The model under review builds one solid part; all positions refer to its coordinate system, in mm. A direction names the side the tool comes from. Round coordinates to 2 decimals unless told otherwise and drop trailing zeros. Order: outer loops, then holes, each group sorted by start corner. A loop starts at its lowest first (then second) coordinate and runs counter-clockwise, first axis right, second up.
1) To check wall thickness, follow L1, parallel to Z at x = 5.75, y = 24 (3 decimals); L2, parallel to X at y = 8, z = -2.5. State the ranges of each line that lie inside material, in increasing order.
2) Consider section D-D (y = 18.5). Give the boundary of the cut face in (x, z) (3 decimals).
3) Consider section B-B (x = 9). Give the boundary of the cut face in (y, z) (3 decimals), then the cut area to 3 significant figures.
4) Consider section A-A (y = 30). Give the boundary of the cut face in (x, z) (3 decimals), then the cut area to 3 significant figures.
5) Machinability: for faces 4 (the face through (0, 23, -24)), 5 (the face through (-1.565, 19.482, -37.514)), which of the approach directions +Z, -Z, +X, -X, +Y, -Y give a long, thin tool a straight path to every point of the face, cutting with its end or side? Answer none if there is none.
6) Consider section C-C (x = -2). Give the boundary of the cut face in (y, z), then the cut area to 3 significant figures.
7) Mouldability with a two-part tool opening along Y and no side actions: class faces 1 (the face through (-1.364, 18.457, -1.91)), 2 (the face through (-1, 36.404, -19)), 3 (the face through (-1.61, 26.925, -28.237)) as pulls with the +Y half, pulls with the -Y half, needs draft (parallel to the pull), parting line crosses it, or undercut.
8) Clearance check with flat-ended pins moving along their axes: P1, Ø1, axis at y = 24.5, z = -5.5, coming from the -X side; P2, Ø7, axis at x = 9.09, y = 8.5, coming from the -Z side (3 decimals); P3, Ø1.5, axis at y = 5.5, z = -23, coming from the +X side. State where each tip first meets the part, or that it passes through.
from build123d import *

# Parameters (mm, degrees)
BASE_FLANGE1_DEPTH           = 3.175
SKETCH7_R                    = 3.15
CUT_EXTRUDE3_DEPTH           = 10
EDGE_FLANGE1_STRIP_W         = 19.05
EDGE_FLANGE1_STRIP_H         = 3.175
EDGE_FLANGE1_STRIP_CUT_DEPTH = 36.40397533
EDGE_FLANGE1_DEPTH           = 36.40397533
SKETCH12_R                   = 2.65
CUT_EXTRUDE4_DEPTH           = 10


# Sheet-metal steps are written as plain solids
with BuildPart() as part:
    # Sketch2 → Base-Flange1 (new body)
    with BuildSketch(Plane(origin=(0, 0, 0), x_dir=(0, 0, -1), z_dir=(1, 0, 0))):
        with BuildLine():
            Line((0, 0), (0, 36.40397533))
            Line((0, 36.40397533), (49.693245392, 36.40397533))
            Line((49.693245392, 36.40397533), (24.989293369, 2.07924376))
            ThreePointArc((24.989293369, 2.07924376), (23.211005522, 0.550068473), (20.931069251, 0))
            Line((20.931069251, 0), (0, 0))
        make_face()
    extrude(amount=-BASE_FLANGE1_DEPTH)

    # Sketch7 → Cut-Extrude3 (cut)
    with BuildSketch(Plane.ZY.offset(3.175)):
        with Locations((-27.553898694, 30)):
            Circle(SKETCH7_R)
        with Locations((-12.587671369, 10)):
            Circle(SKETCH7_R)
    extrude(amount=-CUT_EXTRUDE3_DEPTH, mode=Mode.SUBTRACT)

    # Edge-Flange1 strip (across the edge) → Edge-Flange1 strip cut (cut)
    with BuildSketch(Plane(origin=(0, 36.40397533, 0), x_dir=(0, 0, -1), z_dir=(0, -1, 0))):
        with Locations((-3.175, -1.5875)):
            Rectangle(EDGE_FLANGE1_STRIP_W, EDGE_FLANGE1_STRIP_H)
    extrude(amount=EDGE_FLANGE1_STRIP_CUT_DEPTH, mode=Mode.SUBTRACT)

    # Edge-Flange1 section (across the edge) → Edge-Flange1 (add)
    with BuildSketch(Plane(origin=(0, 36.40397533, 0), x_dir=(0, 0, -1), z_dir=(0, -1, 0))):
        with BuildLine():
            Line((0, 3.175), (0, 15))
            Line((0, 15), (3.175, 15))
            Line((3.175, 15), (3.175, 3.175))
            ThreePointArc((3.175, 3.175), (4.10493597, 0.92993597), (6.35, 0))
            Line((6.35, 0), (6.35, -3.175))
            ThreePointArc((6.35, -3.175), (1.859871939, -1.315128061), (0, 3.175))
        make_face()
    extrude(amount=EDGE_FLANGE1_DEPTH)

    # Sketch12 → Cut-Extrude4 (cut)
    with BuildSketch(Plane(origin=(0, 0, -3.175), x_dir=(-1, 0, 0), z_dir=(0, 0, -1))):
        with Locations((-9.0875, 28.496416241)):
            Circle(SKETCH12_R)
        with Locations((-9.0875, 8.49661674)):
            Circle(SKETCH12_R)
    extrude(amount=-CUT_EXTRUDE4_DEPTH, mode=Mode.SUBTRACT)


solid = part.part
Answer below:
1. L1: z = -3.175 to 0
1. L2: x = -1.87 to 6.48, 11.69 to 15
2. outline: (-3.175, -36.808) - (0, -36.808) - (0, -6.35) arc R3.175 cw to (3.175, -3.175) - (15, -3.175) - (15, 0) - (3.175, 0) arc R6.35 ccw to (-3.175, -6.35) - close
3. outline: (0, -3.175) - (5.848, -3.175) - (5.848, 0) - (0, 0) - close; (11.145, -3.175) - (25.848, -3.175) - (25.848, 0) - (11.145, 0) - close; (31.145, -3.175) - (36.404, -3.175) - (36.404, 0) - (31.145, 0) - close
3. area: 81.9 mm2
4. outline: (-3.175, -45.084) - (0, -45.084) - (0, -30.704) - (-3.175, -30.704) - close; (-3.175, -24.404) - (0, -24.404) - (0, -6.35) arc R3.175 cw to (3.175, -3.175) - (6.905, -3.175) - (6.905, 0) - (3.175, 0) arc R6.35 ccw to (-3.175, -6.35) - close; (11.27, -3.175) - (15, -3.175) - (15, 0) - (11.27, 0) - close
4. area: 150 mm2
5. face 4: -Z, +X, +Y, -Y
5. face 5: -Z, +X, -X, -Y
6. outline: (0, -20.93) arc R5 ccw to (2.08, -24.99) - (36.4, -49.69) - (36.4, -2.67) - (0, -2.67) - close; hole circle Ø6.3 at (10, -12.59); hole circle Ø6.3 at (30, -27.55)
6. area: 1,170 mm2
7. face 1: needs draft
7. face 2: pulls with the +Y half
7. face 3: undercut
8. P1: stops at x = -3.17
8. P2: stops at z = -3.175
8. P3: stops at x = 0
